CAD build for the part. Positions are in the model's coordinates, mm. Give positions to 0.01 mm unless a question says otherwise; leave off trailing zeros. Order: outer loops, then holes, each group sorted by start corner. A loop starts at its lowest first (then second) coordinate and runs counter-clockwise, first axis right, second up. Notation, with made-up numbers: M 43.25,84.5 L 64.25,84.5 A24 ccw 64.25,98.5 Z; hole C 54.5,-2.75 d6. An arc over 180 degrees is marked long. Put each result on its own line as item: value. Start each with the question number.
1) Cut at D-D (z = -4.75). Write the cut outline in (x, y), and give its area (3 significant figures).
2) Cut at C-C (x = 38). Write the cut outline in (y, z).
3) Drill centre lines: line 1 (Z direction, x = 7.5, y = 22); line 2 (Z direction, x = 26.5, y = 10). Where is each one in solid material? Low to high. Write a range as [from, to].
4) Pin check, flat tips, straight feed: pin 1 (1.8 mm diameter, centred on x = 34, z = -11.5, fed in from +Y); pin 2 (4 mm diameter, centred on x = 33.59, z = -11.32, fed in from -Y); pin 3 (1 mm diameter, centred on x = 35, z = -7, fed in from +Y); pin 4 (4 mm diameter, centred on x = 35.5, y = 11.5, fed in from -Z). Stop position of each tip, or through.
5) Cut at A-A (y = 43). Give the number of separate pieces and of enclosed holes in the cut face, and give its area (3 significant figures).
Autodesk Inventor part; units mm, degrees
ref_plane "YZ Plane" through (0, 0, 0) normal (1, 0, 0) x (0, 1, 0)
ref_plane "XZ Plane" through (0, 0, 0) normal (0, 1, 0) x (-1, 0, 0)
ref_plane "XY Plane" through (0, 0, 0) normal (0, 0, 1) x (1, 0, 0)
sketch "Эскиз1" plane through (0, 0, 0) normal (0, 1, 0) x (-1, 0, 0)
  line L0 (-53.5804, -13.9309) -> (-0.75, -0.195)
  line L1 (-52.3223, -18.77) -> (-0.75, -5.3612)
  line L2 (-55.3709, -15.7214) -> (-55.3709, -16.9796)
  circle A0 centre (-52.9514, -16.3505) radius 1.65
  line L3 (-0.75, -5.3612) -> (-0.75, -0.195)
  arc A1 (-55.3709, -16.9796) -> (-52.3223, -18.77) centre (-52.9514, -16.3505) ccw
  arc A2 (-53.5804, -13.9309) -> (-55.3709, -15.7214) centre (-52.9514, -16.3505) ccw
  point P0 (0, 0)
extrude "Выдавливание1" add sketch "Эскиз1" along normal blind 50
sketch "Эскиз24" plane through (0, 50, 0) normal (0, 1, 0) x (1, 0, 0)
  circle A0 centre (52.9514, 16.3505) radius 1.65
  line L0 (52.9514, 16.3505) -> (43.2731, 13.8341)
  circle A1 centre (43.2731, 13.8341) radius 1.65
  circle A2 centre (38.434, 12.576) radius 1.65
  line L1 (48.1122, 15.0923) -> (38.434, 12.576)
  circle A3 centre (33.5949, 11.3178) radius 1.65
  line L2 (43.2731, 13.8341) -> (33.5949, 11.3178)
  circle A4 centre (28.7558, 10.0596) radius 1.65
  line L3 (38.434, 12.576) -> (28.7558, 10.0596)
  circle A5 centre (23.9167, 8.8015) radius 1.65
  line L4 (33.5949, 11.3178) -> (23.9167, 8.8015)
  circle A6 centre (19.0776, 7.5433) radius 1.65
  line L5 (28.7558, 10.0596) -> (19.0776, 7.5433)
  point P0 (0, 0)
  dimension "d126" = 3.3
  dimension "d129" = 5
extrude "Выдавливание24" cut sketch "Эскиз24" against normal blind 3 contours A6 | A5 L5 L4 | L4 L5 A5 | A4 L4 L3 | L3 L4 A4 | A3 L3 L2 | L2 L3 A3 | A2 L2 L1 | L1 L2 A2 | A1 L1 L0 | L0 L1 A1
sketch "Эскиз25" plane through (19.0776, 47, -7.5433) normal (0, 1, 0) x (1, 0, 0)
  circle A0 centre (0, 0) radius 1.65
  circle A1 centre (0, 0) radius 1.15
  circle A2 centre (4.8391, 1.2582) radius 1.65
  circle A3 centre (4.8391, 1.2582) radius 1.15
  circle A4 centre (9.6782, 2.5163) radius 1.65
  circle A5 centre (9.6782, 2.5163) radius 1.15
  circle A6 centre (14.5173, 3.7745) radius 1.65
  circle A7 centre (14.5173, 3.7745) radius 1.15
  circle A8 centre (19.3565, 5.0327) radius 1.65
  circle A9 centre (19.3565, 5.0327) radius 1.15
  circle A10 centre (24.1956, 6.2908) radius 1.65
  circle A11 centre (24.1956, 6.2908) radius 1.15
  point P0 (-19.0776, -7.5433)
  dimension "d136" = 2.3
  dimension "d137" = 2.3
  dimension "d138" = 2.3
  dimension "d139" = 2.3
  dimension "d140" = 2.3
  dimension "d141" = 2.3
extrude "Выдавливание25" cut sketch "Эскиз25" against normal blind 5 contours A1 | A3 | A5 | A7 | A9 | A11
properties part number "only_gate"
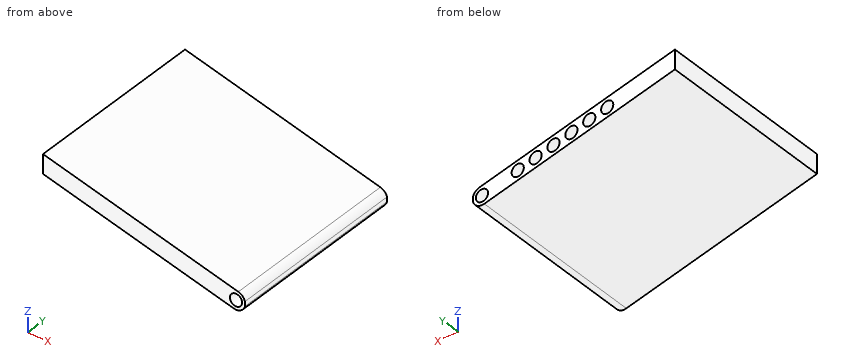
Solution:
1. outline: M 0.75,0 L 18.27,0 L 18.27,50 L 0.75,50 Z
1. area: 876 mm²
2. outline: M 0,-15.05 L 50,-15.05 L 50,-14.17 L 47,-14.17 L 47,-13.64 L 42,-13.64 L 42,-11.51 L 47,-11.51 L 47,-10.98 L 50,-10.98 L 50,-9.88 L 0,-9.88 Z
3. line 1: [-7.12, -1.95]
3. line 2: [-12.06, -6.89]
4. pin 1: y = 47
4. pin 2: y = 0
4. pin 3: through
4. pin 4: z = -14.92
5. separate pieces: 1
5. enclosed holes: 7
5. area: 246 mm²
